Build history of the part. All positions in model axes, mm. Face numbers are marked on the shaded views. A direction names the side the tool comes from. Coordinates: 2 decimals unless noted, no trailing zeros. Order: outer loops, then holes, each group sorted by start corner. A loop starts at its lowest first (then second) coordinate and runs counter-clockwise, first axis right, second up. Notation, with made-up numbers: M 15,59 L 26,59 A17 ccw 26,89 Z; hole C 30.5,34.5 d1. An arc over 180 degrees is marked long. Write item = value, one per line. Start each with the question number.
Q1. Band-saw the part on A-A on x = 0. State how many separate pieces and enclosed holes the cut face has, plus the area to 3 significant figures.
Q2. Drill centre lines: probe 1 along Z at (x, y) = (6.5, 18); probe 2 along X at (y, z) = (0.5, 10.5); probe 3 along Y at (x, z) = (6.5, 13). Where is each one in solid material? Low to high.
Q3. 3-axis set-ups, long thin cutter, end or side, ignore diameter. For the marked faces 1 and 2: which of +Z, -Z, +X, -X, +Y, -Y reach the whole face in a straight line?
Q4. Band-saw the part on D-D on z = 5. Write the cut outline in (x, y).
Q5. Pull direction X, two halves, no side cores. Call the marked faces 3, 4 and 5: released by +X, released by -X, zero draft, split by the parting line, or undercut.
Q6. Pin check, flat tips, straight feed: P1, Ø3.5, axis at x = -23.37, y = 0, coming from the +Z side; P2, Ø10, axis at x = -7.5, z = 12.5, coming from the -Y side; P3, Ø9.5, axis at x = 0, z = 6.77, coming from the -Y side; P4, Ø1.5, axis at x = 7, z = 13.5, coming from the -Y side. Stop position of each tip, or through.
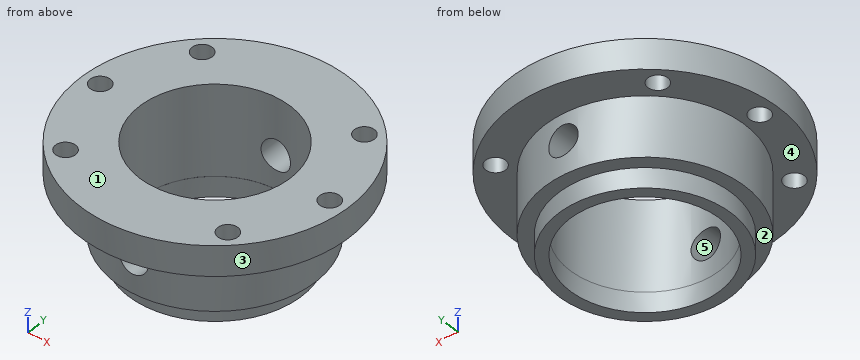
```python
from build123d import *

# Parameters (mm, degrees)
SKETCH_1_R          = 26.8
SKETCH_1_R_2        = 15
EXTRUDE_1_DEPTH     = 18
SKETCH_2_R          = 17.253
SKETCH_2_R_2        = 14.981500248
EXTRUDE_2_DEPTH     = 4
SKETCH_3_R          = 26.8
SKETCH_3_R_2        = 19.94
CUT_EXTRUDE_3_DEPTH = 12
SKETCH_5_R          = 2
CUT_EXTRUDE_4_DEPTH = 42.139761788
SKETCH_7_R          = 3
CUT_EXTRUDE_8_DEPTH = 100


with BuildPart() as part:
    # Эскиз1 → Вытянуть1 (new body)
    with BuildSketch(Plane.XY):
        Circle(SKETCH_1_R)
        Circle(SKETCH_1_R_2, mode=Mode.SUBTRACT)
    extrude(amount=EXTRUDE_1_DEPTH)

    # Эскиз2 → Вытянуть2 (add)
    with BuildSketch(Plane(origin=(0, 0, 0), x_dir=(-1, 0, 0), z_dir=(0, 0, -1))):
        with Locations(Location((0, 0, 0), (0, 0, 180))):
            Circle(SKETCH_2_R)
        Circle(SKETCH_2_R_2, mode=Mode.SUBTRACT)
    extrude(amount=EXTRUDE_2_DEPTH)

    # Эскиз3 → Вытянуть3 (cut)
    with BuildSketch(Plane(origin=(0, 0, 0), x_dir=(-1, 0, 0), z_dir=(0, 0, -1))):
        Circle(SKETCH_3_R)
        Circle(SKETCH_3_R_2, mode=Mode.SUBTRACT)
    extrude(amount=-CUT_EXTRUDE_3_DEPTH, mode=Mode.SUBTRACT)

    # Эскиз5 → Вытянуть4 (cut, through all)
    with BuildSketch(Plane(origin=(0, 0, 12), x_dir=(-1, 0, 0), z_dir=(0, 0, -1))):
        with Locations((-23.37, 0)):
            Circle(SKETCH_5_R)
        with Locations((-16.525085476, 16.525085476)):
            Circle(SKETCH_5_R)
        with Locations((16.525085476, 16.525085476)):
            Circle(SKETCH_5_R)
        with Locations((23.37, 0)):
            Circle(SKETCH_5_R)
        with Locations((16.525085476, -16.525085476)):
            Circle(SKETCH_5_R)
        with Locations((-16.525085476, -16.525085476)):
            Circle(SKETCH_5_R)
    extrude(amount=-CUT_EXTRUDE_4_DEPTH, mode=Mode.SUBTRACT)

    # Эскиз7 → Вытянуть8 (cut)
    with BuildSketch(Plane(origin=(0, 29.05014473, 12), x_dir=(1, 0, 0), z_dir=(0, -1, 0))):
        with Locations(Location((0, -5.233499887, 0), (0, 0, 90))):
            Circle(SKETCH_7_R)
    extrude(amount=CUT_EXTRUDE_8_DEPTH, mode=Mode.SUBTRACT)


solid = part.part
```
Recorded:
q1.separate_pieces = 4
q1.enclosed_holes = 0
q1.area = 219 mm2
q2.probe_1 = 0 to 18
q2.probe_2 = -19.93 to -14.99, 14.99 to 19.93
q2.probe_3 = -26 to -13.52, 13.52 to 26
q3.face_1 = +Z, +X, -X, +Y, -Y
q3.face_2 = -Z
q4.outline = M -2.42,-19.79 L -2.42,-14.8 A15 cw -2.42,14.8 L -2.42,19.79 A19.94 ccw Z; M 2.42,-19.79 A19.94 ccw 2.42,19.79 L 2.42,14.8 A15 cw 2.42,-14.8 Z
q5.face_3 = split by the parting line
q5.face_4 = zero draft
q5.face_5 = undercut
q6.P1 = through
q6.P2 = -26.68
q6.P3 = -19.94
q6.P4 = -26.06
